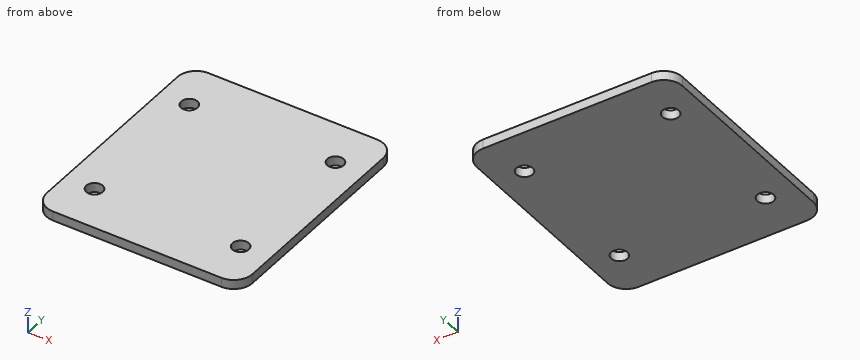
Autodesk Fusion 360 part; units mm, degrees
sketch "Sketch1" plane through (0, 0, 0) normal (0, 0, 1) x (1, 0, 0)
  line L0 (22, 25) -> (-22, 25)
  line L1 (-22, 25) -> (-22, -25)
  line L2 (-22, -25) -> (22, -25)
  line L3 (22, -25) -> (22, 25)
  line L4 (22, 25) -> (-22, -25) construction
  line L5 (-22, 25) -> (22, -25) construction
  line L6 (18.6, 18.6) -> (-18.6, 18.6)
  line L7 (-18.6, 18.6) -> (-18.6, -18.6)
  line L8 (-18.6, -18.6) -> (18.6, -18.6)
  line L9 (18.6, -18.6) -> (18.6, 18.6)
  line L10 (18.6, 18.6) -> (-18.6, -18.6) construction
  line L11 (-18.6, 18.6) -> (18.6, -18.6) construction
  line L12 (-18.6, 18.6) -> (-15.6272, 15.2218)
  circle A0 centre (-15.6272, 15.2218) radius 1.75
  line L13 (0, -25) -> (0, 25)
  line L14 (22, 0) -> (-22, 0)
  circle A1 centre (-15.6272, -15.2218) radius 1.75
  circle A2 centre (15.6272, -15.2218) radius 1.75
  circle A3 centre (15.6272, 15.2218) radius 1.75
  line L15 (-15.6272, 15.2218) -> (-18.6, 15.2218)
  line L16 (-18.6, 15.2218) -> (-22, 15.2218)
  line L17 (-18.8272, 15.2218) -> (-17.2272, 12.4505)
  line L18 (-17.2272, 12.4505) -> (-14.0272, 12.4505)
  line L19 (-14.0272, 12.4505) -> (-12.4272, 15.2218)
  line L20 (-12.4272, 15.2218) -> (-14.0272, 17.9931)
  line L21 (-14.0272, 17.9931) -> (-17.2272, 17.9931)
  line L22 (-17.2272, 17.9931) -> (-18.8272, 15.2218)
  line L23 (14.0272, 12.4505) -> (12.4272, 15.2218)
  line L24 (12.4272, 15.2218) -> (14.0272, 17.9931)
  line L25 (14.0272, 17.9931) -> (17.2272, 17.9931)
  line L26 (17.2272, 17.9931) -> (18.8272, 15.2218)
  line L27 (18.8272, 15.2218) -> (17.2272, 12.4505)
  line L28 (17.2272, 12.4505) -> (14.0272, 12.4505)
  line L29 (-14.0272, -17.9931) -> (-17.2272, -17.9931)
  line L30 (-17.2272, -17.9931) -> (-18.8272, -15.2218)
  line L31 (-12.4272, -15.2218) -> (-14.0272, -17.9931)
  line L32 (-14.0272, -12.4505) -> (-12.4272, -15.2218)
  line L33 (-17.2272, -12.4505) -> (-14.0272, -12.4505)
  line L34 (-18.8272, -15.2218) -> (-17.2272, -12.4505)
  line L35 (18.8272, -15.2218) -> (17.2272, -12.4505)
  line L36 (17.2272, -17.9931) -> (18.8272, -15.2218)
  line L37 (14.0272, -17.9931) -> (17.2272, -17.9931)
  line L38 (12.4272, -15.2218) -> (14.0272, -17.9931)
  line L39 (14.0272, -12.4505) -> (12.4272, -15.2218)
  line L40 (17.2272, -12.4505) -> (14.0272, -12.4505)
  point P0 (-15.6272, 15.2218)
  dimension "d1" = 44
  dimension "d2" = 50
  dimension "d3" = 37.2
  dimension "d4" = 37.2
  dimension "d5" = 4.5
  dimension "d6" = 3.5
  dimension "d11" = 3.2
extrude "Extrude1" add sketch "Sketch1" along normal blind 2 contours L0 L3 L6 L9 L13 L14 L26 L27 | L0 L1 L6 L7 L13 L16 L22 | L2 L3 L8 L9 L13 L14 L35 L36 | L6 L7 L12 L13 L14 L17 L18 L19 L20 L21 L22 | L6 L9 L13 L14 L23 L24 L25 L26 L27 L28 | L8 L9 L13 L14 L35 L36 L37 L38 L39 L40 | L1 L7 L14 L16 L17 | L7 L12 L22 | L7 L8 L13 L14 L29 L30 L31 L32 L33 L34 | L1 L2 L7 L8 L13 L14 L30 L34 | L9 L35 L36 | L9 L35 L36 L37 L38 L39 L40 | L9 L23 L24 L25 L26 L27 L28 | L9 L26 L27 | L7 L16 L22 | L7 L16 L17 | L7 L12 A0 L15 L22 | L7 L12 A0 L15 L17 L18 L19 L20 L21 L22 | L7 L29 L30 L31 L32 L33 L34 | L7 L30 L34
fillet "Fillet1" radius 4 4 edges at (22, -25, 1) (-22, -25, 1) (-22, 25, 1) (22, 25, 1)
The model under review builds one solid part; all positions refer to its coordinate system, in mm. Round coordinates to 2 decimals unless told otherwise and drop trailing zeros. Write each loop counter-clockwise with the first axis right and the second up, starting at its lowest first coordinate (ties: lowest second). Pieces come first, ordered by that corner, then holes. Notation, with made-up numbers: (54, -24.75) - (63, -24.75) arc R38 ccw to (63, 13.25) - close; hole circle Ø2 at (-12, 88). An arc over 180 degrees is marked (long way). One line per item, written item: value. Start each with the question number.
1. Consider section A-A on x = 16.5. Write out the cut boundary in (y, z).
2. Consider section B-B on z = 1.6. Write out the cut boundary in (x, y), and give its area (3 significant figures).
3. To check wall thickness, follow L1, parallel to Y at x = 15.5, z = 1.8; L2, parallel to X at y = -15.5, z = 0.1; L3, parallel to Y at x = 15, z = 1.15. State the ranges of each line that lie inside material, in increasing order. Write a range as from..to.
Checks:
1. outline: (-25, 0) - (-16.74, 0) - (-16.74, 2) - (-25, 2) - close; (-13.7, 0) - (13.7, 0) - (13.7, 2) - (-13.7, 2) - close; (16.74, 0) - (25, 0) - (25, 2) - (16.74, 2) - close
2. outline: (-22, -21) arc R4 ccw to (-18, -25) - (18, -25) arc R4 ccw to (22, -21) - (22, 21) arc R4 ccw to (18, 25) - (-18, 25) arc R4 ccw to (-22, 21) - close; hole circle Ø3.5 at (-15.63, -15.22); hole circle Ø3.5 at (-15.63, 15.22); hole circle Ø3.5 at (15.63, -15.22); hole circle Ø3.5 at (15.63, 15.22)
2. area: 2,150 mm^2
3. L1: y = -25..-16.97, -13.48..13.48, 16.97..25
3. L2: x = -22..-17.35, -13.9..13.9, 17.35..22
3. L3: y = -25..-16.86, -13.59..13.59, 16.86..25
